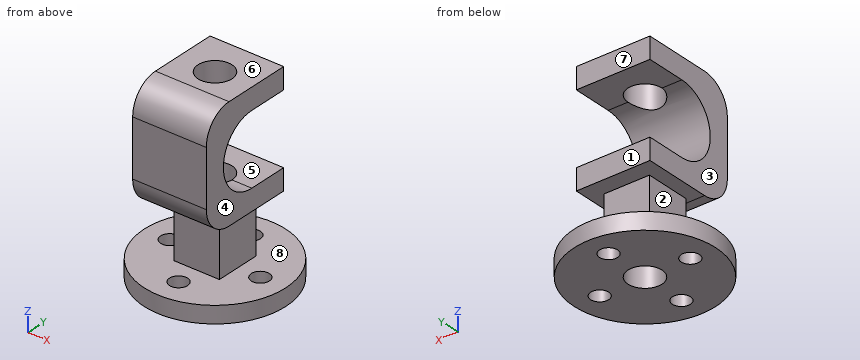
from build123d import *

# Parameters (mm, degrees)
SKETCH_1_R          = 12.5
SKETCH_1_R_2        = 1.6
EXTRUDE_1_DEPTH     = 3
SKETCH_2_W          = 8
SKETCH_2_H          = 8
EXTRUDE_2_DEPTH     = 10
EXTRUDE_3_DEPTH     = 6.5
SKETCH_5_R          = 3
CUT_EXTRUDE_1_DEPTH = 38.436613095
FILLET_1_R          = 5


with BuildPart() as part:
    # 草图1 → 凸台-拉伸1 (new body)
    with BuildSketch(Plane.XY):
        Circle(SKETCH_1_R)
        with Locations((0, 8)):
            Circle(SKETCH_1_R_2, mode=Mode.SUBTRACT)
        with Locations((8, 0)):
            Circle(SKETCH_1_R_2, mode=Mode.SUBTRACT)
        with Locations((0, -8)):
            Circle(SKETCH_1_R_2, mode=Mode.SUBTRACT)
        with Locations((-8, 0)):
            Circle(SKETCH_1_R_2, mode=Mode.SUBTRACT)
    extrude(amount=EXTRUDE_1_DEPTH)

    # 草图2 → 凸台-拉伸2 (add)
    with BuildSketch(Plane.XY.offset(3)):
        Rectangle(SKETCH_2_W, SKETCH_2_H)
    extrude(amount=EXTRUDE_2_DEPTH)

    # 草图4 → 凸台-拉伸3 (add, symmetric)
    with BuildSketch(Plane.ZY):
        with BuildLine():
            Line((13, -10), (33, -10))
            Line((33, -10), (33, 7))
            Line((33, 7), (29.25, 7))
            Line((29.25, 7), (29.25, 0))
            ThreePointArc((29.25, 0), (23, -6.25), (16.75, 0))
            Line((16.75, 0), (16.75, 7))
            Line((16.75, 7), (13, 7))
            Line((13, 7), (13, -10))
        make_face()
    extrude(amount=EXTRUDE_3_DEPTH, both=True)

    # 草图5 → 切除-拉伸1 (cut, through all)
    with BuildSketch(Plane(origin=(0, 0, 0), x_dir=(-1, 0, 0), z_dir=(0, 0, -1))):
        Circle(SKETCH_5_R)
    extrude(amount=-CUT_EXTRUDE_1_DEPTH, mode=Mode.SUBTRACT)

    # 圆角1
    fillet_1_edges = [part.edges().sort_by_distance(p)[0] for p in [
        (0, -10, 13),
        (0, -10, 33),
    ]]
    fillet(fillet_1_edges, radius=FILLET_1_R)


solid = part.part
Could you check a few things on this model? Use its own coordinates, in mm. Face numbers are marked on the shaded views. A direction names the side the tool comes from. Round coordinates to 2 decimals unless told otherwise and drop trailing zeros. Loops run counter-clockwise (first coordinate to the right, second up) from the corner with the lowest first, then second, coordinate; pieces in that order, holes last. Notation, with made-up numbers: (31, 77.5) -> (47, 77.5) arc R21 cw to (47, 98.5) -> close; hole circle Ø4 at (-24, 51.5). An arc over 180 degrees is marked (long way). Use CSV: the item, a comma, the result in double quotes.
(1) Suppose I cut it at D-D on z = 15.5. Write out the boundary of the cut face in (x, y), plus the area to 3 significant figures.
Return value:
outline,"(-6.5, -9.33) -> (6.5, -9.33) -> (6.5, 7) -> (-6.5, 7) -> close; hole circle Ø6 at (0, 0)"
area,"184 mm²"
(2) Suppose I cut it at C-C on x = 5. Write out the boundary of the cut face in (y, z), plus the area to 3 significant figures.
Return value:
outline,"(-11.46, 0) -> (11.46, 0) -> (11.46, 3) -> (-11.46, 3) -> close; (-10, 18) arc R5 ccw to (-5, 13) -> (7, 13) -> (7, 16.75) -> (0, 16.75) arc R6.25 cw to (0, 29.25) -> (7, 29.25) -> (7, 33) -> (-5, 33) arc R5 ccw to (-10, 28) -> close"
area,"249 mm²"
(3) If we mould it in two halves opening along Z, with no side actions, what happens to the marked faces 6, 7 and 8? For each: +Z half, -Z half, draft (parallel to the pull), parting line (faces both ways), or undercut.
Return value:
face 6,"+Z half"
face 7,"draft"
face 8,"undercut"
(4) Suppose I cut it at B-B on x = -2.5. Write out the boundary of the cut face in (y, z).
Return value:
outline,"(-12.25, 0) -> (-1.66, 0) -> (-1.66, 16.97) arc R6.25 cw to (-1.66, 29.03) -> (-1.66, 33) -> (-5, 33) arc R5 ccw to (-10, 28) -> (-10, 18) arc R5 ccw to (-5, 13) -> (-4, 13) -> (-4, 3) -> (-12.25, 3) -> close; (1.66, 0) -> (12.25, 0) -> (12.25, 3) -> (4, 3) -> (4, 13) -> (7, 13) -> (7, 16.75) -> (1.66, 16.75) -> close; (1.66, 29.25) -> (7, 29.25) -> (7, 33) -> (1.66, 33) -> close"
(5) Will these pins go through, and if not, where does the flat tip stop? pin 1 Ø4 at (x, z) = (1.5, 14.5) entering from +Y; pin 2 Ø6 at (x, y) = (-2, 1) entering from +Z; pin 3 Ø5 at (x, z) = (-5.5, 21) entering from +Y; pin 4 Ø2.5 at (y, z) = (0.5, 9.5) entering from +X.
Return value:
pin 1,"stops at y = 7"
pin 2,"stops at z = 33"
pin 3,"stops at y = -4.34"
pin 4,"stops at x = 4"
(6) For the marked faces 1, 2, 3, 4 and 5, which set-ups out of +Z, -Z, +X, -X, +Y, -Y let a thin tool reach every point of the face, with its end or its side?
Return value:
face 1,"+Z, +X, -X, +Y"
face 2,"-X, +Y, -Y"
face 3,"+Z, -X, +Y, -Y"
face 4,"+Z, +X, +Y, -Y"
face 5,"+X, -X, +Y"
(7) Suppose I cut it at A-A on x = 0. Give the number of separate pieces and of enclosed holes in the cut face, plus the area to 3 significant figures.
Return value:
separate pieces,"5"
enclosed holes,"0"
area,"192 mm²"
(8) If I drill on probe 1 along Y at (x, z) = (0, 2); probe 2 along Z at (x, y) = (3, 2); probe 3 along Z at (x, y) = (0, 5.75), over which ranges is the centre line in solid material (lowest first)? Write a range as [from, to].
Return value:
probe 1,"y = [-12.5, -9.6], [-6.4, -3], [3, 6.4], [9.6, 12.5]"
probe 2,"z = [0, 16.75], [29.25, 33]"
probe 3,"z = [0, 3], [13, 16.75], [29.25, 33]"
